Source: three-view drawing plus pictorial views. Frame: mm from the lowest corner of the part. A direction names the side the tool comes from. Give positions to 0.01 mm unless a question says otherwise; leave off trailing zeros. Write each loop counter-clockwise with the first axis right and the second up, starting at its lowest first coordinate (ties: lowest second). Pieces come first, ordered by that corner, then holes. Notation, with made-up numbers: (10, -1) -> (65, -1) arc R12 cw to (65, 11) -> close; hole circle Ø3 at (-39.5, 49). An arc over 180 degrees is marked (long way). Write item = value, one per line.
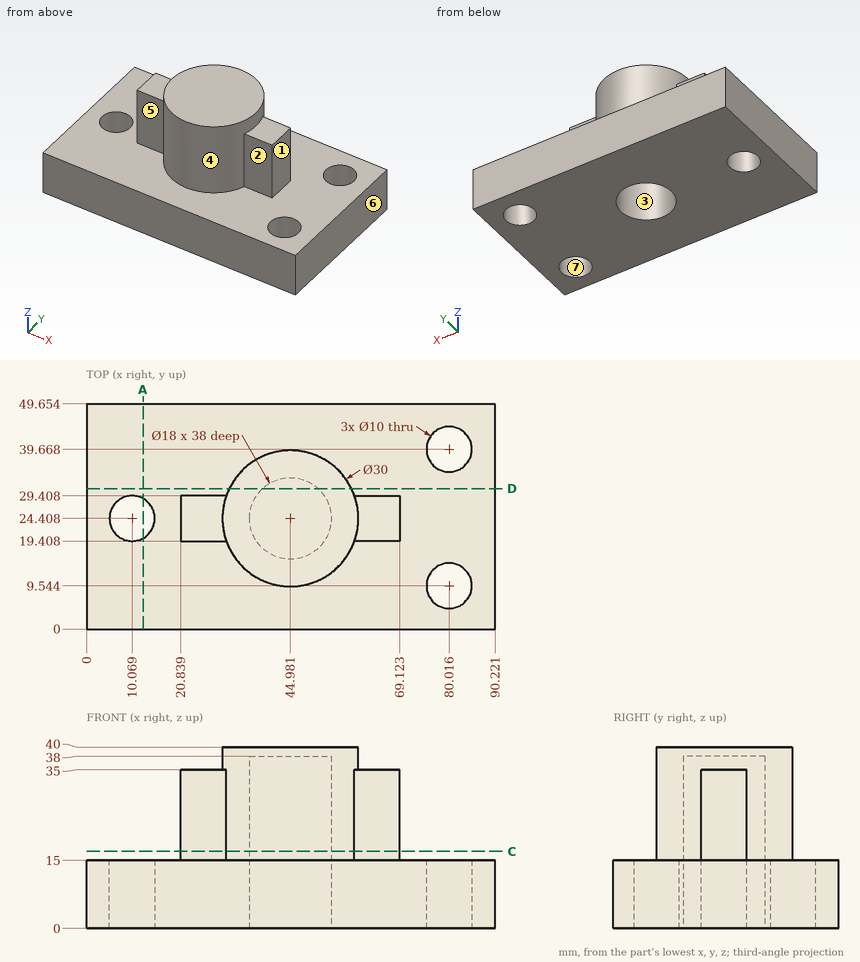
1) Material intervals for L1, parallel to Z at x = 14.5, y = 4.5; L2, parallel to Y at x = 48, z = 13 (1 decimal); L3, parallel to X at y = 23.5, z = 22 (1 decimal), sorted ascending.
Computed:
L1 = 0 to 15
L2 = 0 to 15.9, 32.9 to 49.7
L3 = 20.8 to 36, 53.9 to 69.1
2) Cut plane D-D (y = 31). Return the cut outline in (x, z) (1 decimal).
Computed:
outline = (0, 0) -> (38.9, 0) -> (38.9, 38) -> (51.1, 38) -> (51.1, 0) -> (90.2, 0) -> (90.2, 15) -> (58.5, 15) -> (58.5, 40) -> (31.5, 40) -> (31.5, 15) -> (0, 15) -> close
3) Draft query along Y for the marked faces 5, 6 and 7. Return one class per face: pulls with the +Y half, pulls with the -Y half, needs draft (parallel to the pull), parting line crosses it, or undercut.
Computed:
face_5 = pulls with the -Y half
face_6 = needs draft
face_7 = undercut
4) Contact query for flat-ended pins moving along their axis: pin 1 (14.5 mm diameter, centred on x = 45.5, y = 28.5, fed in from -Z); pin 2 (3 mm diameter, centred on y = 23.5, z = 29.5, fed in from +X); pin 3 (5 mm diameter, centred on y = 23.5, z = 20.5, fed in from -X); pin 4 (4 mm diameter, centred on x = 21.5, z = 21.5, fed in from +Y). Output: stop coordinate, or through.
Computed:
pin_1 = 0
pin_2 = 69.12
pin_3 = 20.84
pin_4 = 29.41
5) Cut plane A-A (x = 12.5). Return the cut outline in (y, z).
Computed:
outline = (0, 0) -> (20.04, 0) -> (20.04, 15) -> (0, 15) -> close; (28.78, 0) -> (49.65, 0) -> (49.65, 15) -> (28.78, 15) -> close
6) Access query for the marked faces 1, 2, 3 and 4. Directions: +Z, -Z, +X, -X, +Y, -Y. A direction counts if a zero-diameter tool reaches every point of the face in a straight line with its end or side. Return the directions, or none.
Computed:
face_1 = +Z, +X, +Y, -Y
face_2 = +Z, +X, -Y
face_3 = -Z
face_4 = +Z
7) Cut plane C-C (z = 17). Return the cut outline in (x, y), then the cut area to 3 significant figures.
Computed:
outline = (20.84, 19.41) -> (30.84, 19.41) arc R15 ccw to (59.12, 19.41) -> (69.12, 19.41) -> (69.12, 29.41) -> (59.12, 29.41) arc R15 ccw to (30.84, 29.41) -> (20.84, 29.41) -> close; hole circle Ø18 at (44.98, 24.41)
area = 641 mm²
